```python
from build123d import *

# Parameters (mm, degrees)
ESQUISSE1_W        = 34
ESQUISSE1_H        = 100.65
BOSS_EXTRU_1_DEPTH = 1.5
ESQUISSE2_W        = 30.8
ESQUISSE2_H        = 97.45
ESQUISSE2_W_2      = 28
ESQUISSE2_H_2      = 94.65
BOSS_EXTRU_2_DEPTH = 1.4
CONG_6_R           = 2
CONG_8_R           = 2
CONG_9_R           = 2


with BuildPart() as part:
    # Esquisse1 → Boss.-Extru.1 (new body)
    with BuildSketch(Plane.XY):
        with Locations((17, 50.325)):
            Rectangle(ESQUISSE1_W, ESQUISSE1_H)
    extrude(amount=BOSS_EXTRU_1_DEPTH)

    # Esquisse2 → Boss.-Extru.2 (add)
    with BuildSketch(Plane.XY.offset(1.5)):
        with Locations((17, 50.325)):
            Rectangle(ESQUISSE2_W, ESQUISSE2_H)
        with Locations((17, 50.325)):
            Rectangle(ESQUISSE2_W_2, ESQUISSE2_H_2, mode=Mode.SUBTRACT)
    extrude(amount=BOSS_EXTRU_2_DEPTH)

    # Congé6
    cong_6_edges = [part.edges().sort_by_distance(p)[0] for p in [
        (0, 0, 0.75),
    ]]
    fillet(cong_6_edges, radius=CONG_6_R)

    # Congé8
    cong_8_edges = [part.edges().sort_by_distance(p)[0] for p in [
        (0, 100.65, 0.75),
    ]]
    fillet(cong_8_edges, radius=CONG_8_R)

    # Congé9
    # the kernel refuses this fillet: 2 mm, written as the material it takes off along each edge
    with BuildSketch(Plane(origin=(38.841229183, 100.65, 0), x_dir=(0, -1, 0), z_dir=(-1, 0, 0)), Plane(origin=(2, 0, 0), x_dir=(0, 1, 0), z_dir=(1, 0, 0))) as cong_9_piece_1:
        with BuildLine():
            CenterArc((1.936491673, 2), CONG_9_R, 194.477512186, 75.522487814)
            Line((0, 1.5), (-0.038729833, 1.49))
            ThreePointArc((-0.038729833, 1.49), (-0.04, 0.75), (-0.04, 0))
            Line((-0.04, 0), (0, -0.04))
            Line((0, -0.04), (1.936491673, -0.04))
            Line((1.936491673, -0.04), (1.936491673, 0))
        make_face()
    extrude(amount=36.841229183, mode=Mode.SUBTRACT)
    with BuildSketch(Plane(origin=(2, 98.65, 0), x_dir=(-1, 0, 0), z_dir=(0, -1, 0))) as cong_9_piece_2:
        with BuildLine():
            CenterArc((0.063508327, -2), CONG_9_R, 14.477512186, 75.522487814)
            Line((2, -1.5), (2.038729833, -1.49))
            ThreePointArc((2.038729833, -1.49), (2.04, -0.75), (2.04, 0))
            Line((2.04, 0), (2, 0.04))
            Line((2, 0.04), (0.063508327, 0.04))
            Line((0.063508327, 0.04), (0.063508327, 0))
        make_face()
    revolve(axis=Axis((2, 98.65, 0), (0, 0, -1)), revolution_arc=90, mode=Mode.SUBTRACT)
    with BuildSketch(Plane(origin=(0, 98.65, 0), x_dir=(1, 0, 0), z_dir=(0, -1, 0))) as cong_9_piece_3:
        with BuildLine():
            CenterArc((1.936491673, 2), CONG_9_R, 194.477512186, 75.522487814)
            Line((0, 1.5), (-0.038729833, 1.49))
            ThreePointArc((-0.038729833, 1.49), (-0.04, 0.75), (-0.04, 0))
            Line((-0.04, 0), (0, -0.04))
            Line((0, -0.04), (1.936491673, -0.04))
            Line((1.936491673, -0.04), (1.936491673, 0))
        make_face()
    extrude(amount=96.65, mode=Mode.SUBTRACT)
    with BuildSketch(Plane(origin=(2, 2, 0), x_dir=(0, -1, 0), z_dir=(1, 0, 0))) as cong_9_piece_4:
        with BuildLine():
            CenterArc((0.063508327, -2), CONG_9_R, 14.477512186, 75.522487814)
            Line((2, -1.5), (2.038729833, -1.49))
            ThreePointArc((2.038729833, -1.49), (2.04, -0.75), (2.04, 0))
            Line((2.04, 0), (2, 0.04))
            Line((2, 0.04), (0.063508327, 0.04))
            Line((0.063508327, 0.04), (0.063508327, 0))
        make_face()
    revolve(axis=Axis((2, 2, 0), (0, 0, -1)), revolution_arc=90, mode=Mode.SUBTRACT)


solid = part.part
```
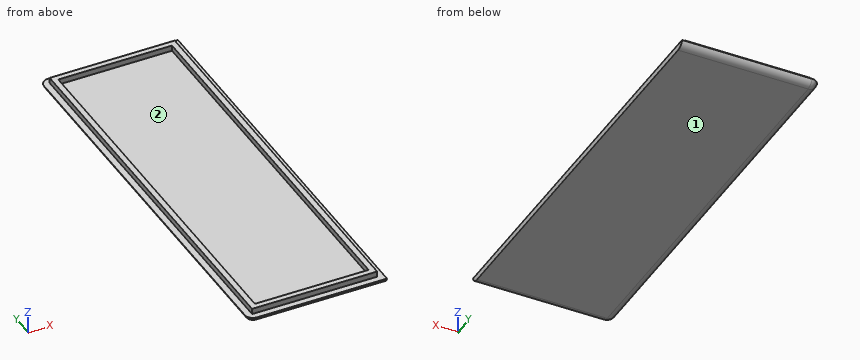
For this review, take the finished solid that the model builds, in its own axes (mm). Face numbers are marked on the shaded views. Coordinates: 2 decimals unless noted, no trailing zeros. Order: outer loops, then holes, each group sorted by start corner. A loop starts at its lowest first (then second) coordinate and runs counter-clockwise, first axis right, second up. Notation, with made-up numbers: (39, -16.75) -> (54, -16.75) arc R13 ccw to (54, 5.25) -> close; hole circle Ø11 at (6, 35.25). An arc over 180 degrees is marked (long way). Use CSV: the item, a comma, the result in double quotes. Start each with the question number.
Item 1: Draft analysis for pull direction Y (two halves, no side actions). For the marked faces 1 and 2, state which applies: pulls with the +Y half, pulls with the -Y half, needs draft (parallel to the pull), parting line crosses it, or undercut.
Item 2: We need section C-C, the plane y = 58. Give the boundary of the cut face in (x, z).
Item 3: We need section B-B, the plane x = 11. Give the boundary of the cut face in (y, z), then the cut area to 3 significant figures.
Item 4: Insertion check: pin 1 (1.5 mm diameter, centred on y = 44.5, z = 2.5, fed in from +X); pin 2 (1 mm diameter, centred on x = 8.5, z = 0.5, fed in from -Y); pin 3 (0.7 mm diameter, centred on y = 51.5, z = 2, fed in from -X). Each pin has a flat end and moves straight along its axis. Give the tip position at first contact, or say it passes through.
Item 5: Wall thickness on probe 1 along X at (y, z) = (94, 2.1); probe 2 along Y at (x, z) = (5, 2.1); probe 3 along Z at (x, y) = (19, 87.5): over which ranges is each line inside the solid? List them lowest first.
Item 6: We need section A-A, the plane z = 2.15. Give the boundary of the cut face in (x, y).
Derived:
1,face 1,"needs draft"
1,face 2,"undercut"
2,outline,"(0, 1.5) arc R2 ccw to (1.94, 0) -> (34, 0) -> (34, 1.5) -> (32.4, 1.5) -> (32.4, 2.9) -> (31, 2.9) -> (31, 1.5) -> (3, 1.5) -> (3, 2.9) -> (1.6, 2.9) -> (1.6, 1.5) -> close"
3,outline,"(0, 1.5) arc R2 ccw to (1.94, 0) -> (98.71, 0) arc R2 ccw to (100.65, 1.5) -> (99.05, 1.5) -> (99.05, 2.9) -> (97.65, 2.9) -> (97.65, 1.5) -> (3, 1.5) -> (3, 2.9) -> (1.6, 2.9) -> (1.6, 1.5) -> close"
3,area,"153 mm^2"
4,pin 1,"stops at x = 32.4"
4,pin 2,"stops at y = 0.2"
4,pin 3,"stops at x = 1.6"
5,probe 1,"x = 1.6 to 3, 31 to 32.4"
5,probe 2,"y = 1.6 to 3, 97.65 to 99.05"
5,probe 3,"z = 0 to 1.5"
6,outline,"(1.6, 1.6) -> (32.4, 1.6) -> (32.4, 99.05) -> (1.6, 99.05) -> close; hole (3, 3) -> (31, 3) -> (31, 97.65) -> (3, 97.65) -> close"
